Autodesk Inventor part; units mm, degrees
ref_plane "РабПлоскость3" through (0, 15, 0) normal (0, 1, 0) x (1, 0, 0)
ref_plane "РабПлоскость1" through (0, 15, 0) normal (0, 1, 0) x (1, 0, 0)
ref_plane "YZ Plane" through (0, 0, 0) normal (1, 0, 0) x (0, 1, 0)
sketch "Эскиз1" plane through (0, 0, 0) normal (0, 1, 0) x (-1, 0, 0)
  line L0 (0, 0) -> (90, 0)
  line L1 (90, 0) -> (90, -60)
  line L2 (90, -60) -> (0, -60)
  line L3 (0, -60) -> (0, 0)
  line L4 (0, -60) -> (66, -60)
  line L5 (0, -30) -> (66, -30)
  circle A0 centre (66, -30) radius 7.5
  dimension "d0" = 90
  dimension "d1" = 60
  dimension "d67" = 66
  dimension "d68" = 15
extrude "Выдавливание1" add sketch "Эскиз1" along normal blind 15
ref_plane "РабПлоскость3" through (0, 15, 0) normal (0, 1, 0) x (1, 0, 0)
sketch "Эскиз3" plane through (0, 15, 0) normal (0, 1, 0) x (1, 0, 0)
  line L0 (0, 0) -> (0, 60)
  line L1 (0, 30) -> (0, 28)
  line L2 (0, 28) -> (-50, 28)
  line L3 (-50, 28) -> (-50, 32)
  line L4 (-50, 32) -> (0, 32)
  line L5 (0, 32) -> (0, 28)
  point P0 (0, 32)
  dimension "d13" = 2
  dimension "d14" = 50
  dimension "d15" = 4
extrude "Выдавливание3" add sketch "Эскиз3" along normal blind 5
ref_plane "РабПлоскость1" through (0, 15, 0) normal (0, 1, 0) x (1, 0, 0)
sketch "Эскиз6" plane through (0, 15, 0) normal (0, 1, 0) x (1, 0, 0)
  circle A0 centre (-66, 30) radius 7.5
  line L0 (-66, 30) -> (-66, -120)
  line L1 (-150, -120) -> (0, -120)
  line L2 (-66, -120) -> (-66, -100)
  circle A1 centre (-66, -100) radius 10
  circle A2 centre (-66, -100) radius 20
  circle A3 centre (-66, 30) radius 40
  line L3 (-85.7619, -103.0769) -> (-105.5238, 23.8462)
  line L4 (-46.2381, -103.0769) -> (-26.4762, 23.8462)
  line L5 (-66, -100) -> (-66, -40)
  line L6 (-66, -40) -> (-91, -40)
  line L7 (-66, -40) -> (-41, -40)
  circle A4 centre (-91, -40) radius 2.5
  circle A5 centre (-41, -40) radius 2.5
  point P0 (0, 0)
  dimension "d45" = 20
  dimension "d46" = 20
  dimension "d47" = 40
  dimension "d48" = 80
  dimension "d49" = 60
  dimension "d50" = 25
  dimension "d52" = 25
  dimension "d53" = 5
  dimension "d54" = 5
sketch "Эскиз7" plane through (0, 0, 0) normal (1, 0, 0) x (0, 0, -1)
  line L0 (80.2787, 0) -> (80.2787, 15)
  line L1 (60, 15) -> (0, 15)
  line L2 (80.2787, 15) -> (60.2787, 15)
  line L3 (60.2787, 15) -> (0, 15)
  line L4 (0, 0) -> (0, 15)
  line L5 (0, 15) -> (-20, 15)
  line L6 (-20, 15) -> (-20, 0)
  line L7 (-20, 0) -> (0, 0)
  line L8 (-20, 7.5) -> (-14, 7.5)
  line L9 (80.2787, 7.5) -> (74.2787, 7.5)
  arc A0 (74.2787, 4.5) -> (74.2787, 10.5) centre (74.2787, 7.5) ccw
  arc A1 (-14, 10.5) -> (-14, 4.5) centre (-14, 7.5) ccw
  line L10 (60, 0) -> (0, 0)
  line L11 (60, 0) -> (0, 0)
  line L12 (60, 0) -> (60, 15)
  line L13 (60, 0) -> (60, 15)
  line L14 (60, 0) -> (80.2787, 0)
  line L15 (74.2787, 4.5) -> (71.2787, 4.5)
  line L16 (71.2787, 10.5) -> (74.2787, 10.5)
  arc A2 (71.2787, 10.5) -> (71.2787, 4.5) centre (71.2787, 7.5) ccw
  line L17 (-14, 7.5) -> (-12, 7.5)
  arc A3 (-12, 4.5) -> (-12, 10.5) centre (-12, 7.5) ccw
  line L18 (-14, 7.5) -> (-14, 10.5)
  line L19 (-14, 10.5) -> (-12, 10.5)
  line L20 (-14, 4.5) -> (-12, 4.5)
  point P0 (-17, 7.5)
  dimension "d59" = 20
  dimension "d60" = 6
  dimension "d61" = 6
  dimension "d62" = 6
  dimension "d63" = 6
extrude "Выдавливание7" add sketch "Эскиз7" against normal blind 3
properties part number "Стенка энкодера штурвала"
Check sheet for the modelled part. Datum: model origin and axes. Units: mm. A direction names the side the tool comes from. Give positions to 0.01 mm unless a question says otherwise; leave off trailing zeros. Write each loop counter-clockwise with the first axis right and the second up, starting at its lowest first coordinate (ties: lowest second). Pieces come first, ordered by that corner, then holes. Notation, with made-up numbers: (79, -12.75) -> (116, -12.75) arc R27 ccw to (116, 8.25) -> close; hole circle Ø5 at (2.25, 51.5). An arc over 180 degrees is marked (long way). One line per item, written item: value. Start each with the question number.
Item 1: Tool access check on faces 4 (the flat face through (-25, 17, -28)), 5 (the flat face through (-25, 17, -32)), 6 (the flat face through (-46, 7, 0)), 7 (the flat face through (-3, 8, -68)), 8 (the cylindrical face through (-1.5, 7.4, 9)). Record the directions out of +Z, -Z, +X, -X, +Y, -Y that give a thin tool (end or side, any length) a straight path to the whole face; none if there is none.
Item 2: Draft check along Z on faces 1 (the flat face through (-90, 7, -30)), 2 (the cylindrical face through (-60.048, 7.395, -25.436)), 3 (the flat face through (-47, 7, -60)). Enter one of: +Z half, -Z half, draft (parallel to the pull), parting line (faces both ways), or undercut.
Item 3: Section check C-C on y = 2.5. Record the cut outline in (x, z).
Item 4: Section check A-A on z = -30. Record the cut outline in (x, y), then the cut area to 4 significant figures.
Item 5: Gauge pin test, flat ends, axial feed: pin 1 (6 mm diameter, centred on x = -80.5, z = -41, fed in from +Y); pin 2 (10 mm diameter, centred on x = -53, y = 10.5, fed in from +Z); pin 3 (7.5 mm diameter, centred on y = 7, z = -74.5, fed in from -X). Record the tip position at first contact, or that the pin passes through.
Item 6: Material ranges on probe 1 along Z at (x, y) = (-66, 10.25); probe 2 along X at (y, z) = (8.5, -30); probe 3 along Y at (x, z) = (-80.5, -18.5), recorded low to high. Write a range as from..to.
Item 7: Section check D-D on x = -65. Record the cut outline in (y, z), then the cut area to 3 significant figures.
Item 8: Section check B-B on y = 7.5. Record the cut outline in (x, z).
Results list:
1. face 4: +Z, +X, -X, +Y
1. face 5: -Z, +X, -X, +Y
1. face 6: +Z, -X, +Y, -Y
1. face 7: -Z, -X, +Y, -Y
1. face 8: +X, -X
2. face 1: draft
2. face 2: undercut
2. face 3: -Z half
3. outline: (-90, -60) -> (-3, -60) -> (-3, -80.28) -> (0, -80.28) -> (0, 20) -> (-3, 20) -> (-3, 0) -> (-90, 0) -> close; hole circle Ø15 at (-66, -30)
4. outline: (-90, 0) -> (-73.5, 0) -> (-73.5, 15) -> (-90, 15) -> close; (-58.5, 0) -> (0, 0) -> (0, 20) -> (-50, 20) -> (-50, 15) -> (-58.5, 15) -> close
4. area: 1,375 mm²
5. pin 1: y = 15
5. pin 2: z = 0
5. pin 3: x = -3
6. probe 1: -60..-37.5, -22.5..0
6. probe 2: -90..-73.5, -58.5..0
6. probe 3: 0..15
7. outline: (0, -60) -> (15, -60) -> (15, -37.43) -> (0, -37.43) -> close; (0, -22.57) -> (15, -22.57) -> (15, 0) -> (0, 0) -> close
7. area: 677 mm²
8. outline: (-90, -60) -> (-3, -60) -> (-3, -68.28) -> (0, -68.28) -> (0, 9) -> (-3, 9) -> (-3, 0) -> (-90, 0) -> close; (-3, -80.28) -> (0, -80.28) -> (0, -77.28) -> (-3, -77.28) -> close; (-3, 17) -> (0, 17) -> (0, 20) -> (-3, 20) -> close; hole circle Ø15 at (-66, -30)
